Geometry: final body of the model. Coordinates: model frame, mm. Face numbers are marked on the shaded views. A direction names the side the tool comes from. Give positions to 0.01 mm unless a question says otherwise; leave off trailing zeros. Loops run counter-clockwise (first coordinate to the right, second up) from the corner with the lowest first, then second, coordinate; pieces in that order, holes last.
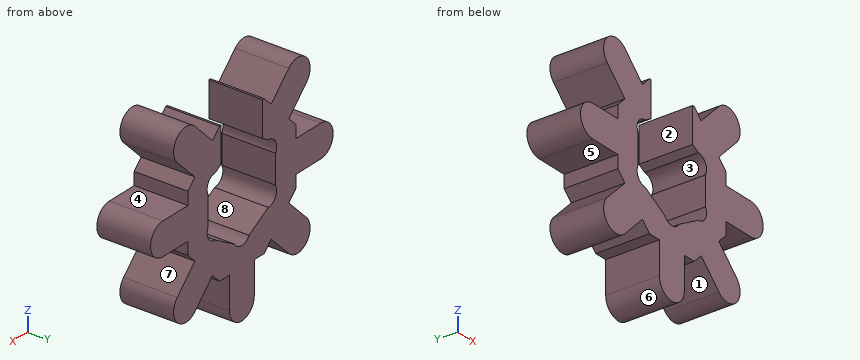
from build123d import *

# Parameters (mm, degrees)
EXTRUDE_2_DEPTH          = 5
CUT_EXTRUDE_1_DEPTH      = 5
SKETCH_5_R               = 1
CUT_EXTRUDE_2_DEPTH      = 5
PATTERN_CIRCULAR_1_COUNT = 6
CUT_EXTRUDE_3_DEPTH      = 10
EXTRUDE_3_DEPTH          = 5


with BuildPart() as part:
    # 스케치3 → 보스-돌출2 (new body)
    with BuildSketch(Plane(origin=(0, 0, 0), x_dir=(1, 0, 0), z_dir=(0, 1, 0))):
        Polygon((2.692388155, 6.5), (-2.692388155, 6.5), (-6.5, 2.692388155), (-6.5, -2.692388155), (-2.692388155, -6.5), (2.692388155, -6.5), (6.5, -2.692388155), (6.5, 2.692388155), align=None)
    extrude(amount=EXTRUDE_2_DEPTH)

    # 스케치4 → 컷-돌출1 (cut)
    with BuildSketch(Plane(origin=(0, 5, 0), x_dir=(1, 0, 0), z_dir=(0, 1, 0))):
        Polygon((4.05, 2.33826859), (0, 4.67653718), (-4.05, 2.33826859), (-4.05, -2.33826859), (0, -4.67653718), (4.05, -2.33826859), align=None)
    extrude(amount=-CUT_EXTRUDE_1_DEPTH, mode=Mode.SUBTRACT)

    # 스케치5 → 컷-돌출2 (cut)
    with BuildSketch(Plane(origin=(0, 5, 0), x_dir=(1, 0, 0), z_dir=(0, 1, 0))):
        with Locations((0, 3.67653718)):
            Circle(SKETCH_5_R)
    cut_extrude_2 = extrude(amount=-CUT_EXTRUDE_2_DEPTH, mode=Mode.SUBTRACT)

    # 원형 패턴1: 컷-돌출2 ×6 about axis
    pattern_circular_1_axis = Axis((0, 0, 0), (0, 1, 0))
    for i in range(1, PATTERN_CIRCULAR_1_COUNT):
        add(cut_extrude_2.rotate(pattern_circular_1_axis, i * 360 / PATTERN_CIRCULAR_1_COUNT), mode=Mode.SUBTRACT)

    # 스케치8 → 컷-돌출3 (cut)
    with BuildSketch(Plane(origin=(0, 5, 0), x_dir=(1, 0, 0), z_dir=(0, 1, 0))):
        with BuildLine():
            Line((2.5, 0), (2.5, -9.615491692))
            ThreePointArc((2.5, -9.615491692), (0, -12.115491692), (-2.5, -9.615491692))
            Line((-2.5, -9.615491692), (-2.5, 0))
            ThreePointArc((-2.5, 0), (0, 2.5), (2.5, 0))
        make_face()
    extrude(amount=-CUT_EXTRUDE_3_DEPTH, mode=Mode.SUBTRACT)

    # 스케치10 → 보스-돌출3 (add)
    with BuildSketch(Plane(origin=(0, 5, 0), x_dir=(1, 0, 0), z_dir=(0, 1, 0))):
        with BuildLine():
            Line((-3.535533906, -5.656854249), (-5.656854249, -7.778174593))
            ThreePointArc((-5.656854249, -7.778174593), (-7.778174593, -7.778174593), (-7.778174593, -5.656854249))
            Line((-7.778174593, -5.656854249), (-5.656854249, -3.535533906))
            ThreePointArc((-5.656854249, -3.535533906), (-3.535533906, -3.535533906), (-3.535533906, -5.656854249))
        make_face()
        with BuildLine():
            Line((-6.5, -1.5), (-9.5, -1.5))
            ThreePointArc((-9.5, -1.5), (-11, 0), (-9.5, 1.5))
            Line((-9.5, 1.5), (-6.5, 1.5))
            ThreePointArc((-6.5, 1.5), (-5, 0), (-6.5, -1.5))
        make_face()
        with BuildLine():
            Line((-5.656854249, 3.535533906), (-7.778174593, 5.656854249))
            ThreePointArc((-7.778174593, 5.656854249), (-7.778174593, 7.778174593), (-5.656854249, 7.778174593))
            Line((-5.656854249, 7.778174593), (-3.535533906, 5.656854249))
            ThreePointArc((-3.535533906, 5.656854249), (-3.535533906, 3.535533906), (-5.656854249, 3.535533906))
        make_face()
        with BuildLine():
            Line((-1.5, 6.5), (-1.5, 9.5))
            ThreePointArc((-1.5, 9.5), (0, 11), (1.5, 9.5))
            Line((1.5, 9.5), (1.5, 6.5))
            ThreePointArc((1.5, 6.5), (0, 5), (-1.5, 6.5))
        make_face()
        with BuildLine():
            Line((3.535533906, 5.656854249), (5.656854249, 7.778174593))
            ThreePointArc((5.656854249, 7.778174593), (7.778174593, 7.778174593), (7.778174593, 5.656854249))
            Line((7.778174593, 5.656854249), (5.656854249, 3.535533906))
            ThreePointArc((5.656854249, 3.535533906), (3.535533906, 3.535533906), (3.535533906, 5.656854249))
        make_face()
        with BuildLine():
            Line((6.5, 1.5), (9.5, 1.5))
            ThreePointArc((9.5, 1.5), (11, 0), (9.5, -1.5))
            Line((9.5, -1.5), (6.5, -1.5))
            ThreePointArc((6.5, -1.5), (5, 0), (6.5, 1.5))
        make_face()
        with BuildLine():
            Line((5.656854249, -3.535533906), (7.778174593, -5.656854249))
            ThreePointArc((7.778174593, -5.656854249), (7.778174593, -7.778174593), (5.656854249, -7.778174593))
            Line((5.656854249, -7.778174593), (3.535533906, -5.656854249))
            ThreePointArc((3.535533906, -5.656854249), (3.535533906, -3.535533906), (5.656854249, -3.535533906))
        make_face()
    extrude(amount=-EXTRUDE_3_DEPTH)


solid = part.part
Item 1: Section query B-B on z = -7. Return loops of the section in (x, y).
Values follow:
outline: (-8.19, 0) - (-4.88, 0) - (-4.88, 5) - (-8.19, 5) - close; (-1.5, 0) - (1.5, 0) - (1.5, 5) - (-1.5, 5) - close; (4.88, 0) - (8.19, 0) - (8.19, 5) - (4.88, 5) - close
Item 2: Section query C-C on x = 6. Return loops of the section in (y, z).
Values follow:
outline: (0, -8.03) - (5, -8.03) - (5, -3.88) - (0, -3.88) - close; (0, -3.19) - (5, -3.19) - (5, 3.19) - (0, 3.19) - close; (0, 3.88) - (5, 3.88) - (5, 8.03) - (0, 8.03) - close
Item 3: Draft query along X for the marked faces 6, 7 and 8. Return one class per face: +X half, -X half, draft (parallel to the pull), parting line (faces both ways), or undercut.
Values follow:
face 6: parting line
face 7: +X half
face 8: undercut
Item 4: Ray query, probe 1 along X at (y, z) = (1.25, -6.75); probe 2 along Z at (x, y) = (-7, 4.05); probe 3 along Z at (x, y) = (8, 4.55). Return the intervals inside material, ascending.
Values follow:
probe 1: x = -8.22 to -4.63, -1.5 to 1.5, 4.63 to 8.22
probe 2: z = -8.19 to -4.88, -1.5 to 1.5, 4.88 to 8.19
probe 3: z = -7.5 to -5.94, -1.5 to 1.5, 5.94 to 7.5
Item 5: Set-up query: the marked faces 1, 2, 3, 4 and 5. Return all of +Z, -Z, +X, -X, +Y, -Y with unobstructed straight access to the full face (end or side cutting, diameter ignored); none if empty.
Values follow:
face 1: -Z, +Y, -Y
face 2: +Z, +Y, -Y
face 3: +Y, -Y
face 4: +X, +Y, -Y
face 5: -X, +Y, -Y
Item 6: Section query A-A on z = 0. Return loops of the section in (x, y).
Values follow:
outline: (-11, 0) - (-4.05, 0) - (-4.05, 5) - (-11, 5) - close; (4.05, 0) - (11, 0) - (11, 5) - (4.05, 5) - close
Item 7: Section query D-D on z = 4.75. Return loops of the section in (x, y).
Values follow:
outline: (-6.87, 0) - (-2.5, 0) - (-2.5, 5) - (-6.87, 5) - close; (2.5, 0) - (6.87, 0) - (6.87, 5) - (2.5, 5) - close
Item 8: Pin query (flat end, axial travel): pin 1 (0.9 mm diameter, centred on y = 2.5, z = -8, fed in from -X); pin 2 (1 mm diameter, centred on y = 3, z = -2.5, fed in from -X); pin 3 (2.5 mm diameter, centred on x = -8, y = 3.5, fed in from -Z). Return the tip coordinate at first contact, or that it passes through.
Values follow:
pin 1: stops at x = -7.97
pin 2: stops at x = -6.5
pin 3: stops at z = -8.22
